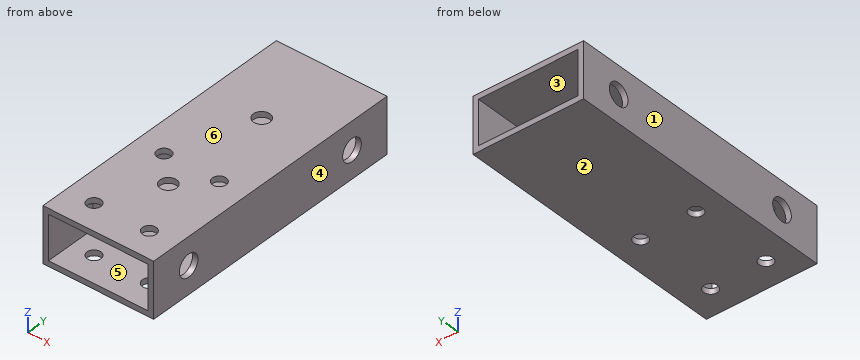
```python
from build123d import *

# Parameters (mm, degrees)
SKICA1_W                 = 40
SKICA1_H                 = 20
SKICA1_W_2               = 36
SKICA1_H_2               = 16
P_IDAT_VYSUNUT_M1_DEPTH  = 100
SKICA2_R                 = 4
ODEBRAT_VYSUNUT_M1_DEPTH = 40
SKETCH1_R                = 2.5
CUT_EXTRUDE1_DEPTH       = 20
SKETCH2_R                = 3
CUT_EXTRUDE2_DEPTH       = 2


with BuildPart() as part:
    # Skica1 → Přidat vysunutím1 (new body)
    with BuildSketch(Plane(origin=(0, 0, 0), x_dir=(1, 0, 0), z_dir=(0, 1, 0))):
        with Locations((20, 10)):
            Rectangle(SKICA1_W, SKICA1_H)
        with Locations((20, 10)):
            Rectangle(SKICA1_W_2, SKICA1_H_2, mode=Mode.SUBTRACT)
    extrude(amount=P_IDAT_VYSUNUT_M1_DEPTH)

    # Skica2 → Odebrat vysunutím1 (cut)
    with BuildSketch(Plane(origin=(40, 0, 0), x_dir=(0, 0, -1), z_dir=(1, 0, 0))):
        with Locations((10, 85)):
            Circle(SKICA2_R)
        with Locations((10, 15)):
            Circle(SKICA2_R)
    extrude(amount=-ODEBRAT_VYSUNUT_M1_DEPTH, mode=Mode.SUBTRACT)

    # Sketch1 → Cut-Extrude1 (cut)
    with BuildSketch(Plane.XY):
        with Locations((10, 10)):
            Circle(SKETCH1_R)
        with Locations((30, 10)):
            Circle(SKETCH1_R)
        with Locations((30, 40)):
            Circle(SKETCH1_R)
        with Locations((10, 40)):
            Circle(SKETCH1_R)
    extrude(amount=-CUT_EXTRUDE1_DEPTH, mode=Mode.SUBTRACT)

    # Sketch2 → Cut-Extrude2 (cut)
    with BuildSketch(Plane.XY):
        with Locations((20, 30)):
            Circle(SKETCH2_R)
        with Locations((20, 70)):
            Circle(SKETCH2_R)
    extrude(amount=-CUT_EXTRUDE2_DEPTH, mode=Mode.SUBTRACT)


solid = part.part
```
Build history of the part. All positions in model axes, mm. Face numbers are marked on the shaded views. A direction names the side the tool comes from. Round coordinates to 2 decimals unless told otherwise and drop trailing zeros. Write each loop counter-clockwise with the first axis right and the second up, starting at its lowest first coordinate (ties: lowest second). Pieces come first, ordered by that corner, then holes.
1) Pin check, flat tips, straight feed: pin 1 (4 mm diameter, centred on x = 10, y = 40, fed in from +Z); pin 2 (5 mm diameter, centred on x = 20, y = 70, fed in from +Z). Stop position of each tip, or through.
2) 3-axis set-ups, long thin cutter, end or side, ignore diameter. For the marked faces 5 and 6: which of +Z, -Z, +X, -X, +Y, -Y reach the whole face in a straight line?
3) Band-saw the part on A-A, the plane z = -5. List the corners of the cut face in (x, y), and give its area (3 significant figures).
4) Drill centre lines: probe 1 along Y at (x, z) = (38.95, -10); probe 2 along X at (y, z) = (37.5, -11.5); probe 3 along Z at (x, y) = (34.5, 90). Where is each one in solid material? Low to high.
5) Mould opens along X. For the marked faces 1, 2, 3 and 4 say: +X half, -X half, draft (parallel to the pull), parting line (faces both ways), or undercut.
6) Band-saw the part on B-B, the plane y = 15. List the corners of the cut face in (x, z), and give its area (3 significant figures).
7) Band-saw the part on C-C, the plane x = 30. List the corners of the cut face in (y, z).
8) Band-saw the part on D-D, the plane x = 20. List the corners of the cut face in (y, z), and give its area (3 significant figures).
Ans:
1. pin 1: passes through
1. pin 2: stops at z = -18
2. face 5: +Y, -Y
2. face 6: +Z, +X, -X, +Y, -Y
3. outline: (0, 0) - (2, 0) - (2, 100) - (0, 100) - close; (38, 0) - (40, 0) - (40, 100) - (38, 100) - close
3. area: 400 mm2
4. probe 1: y = 0 to 11, 19 to 81, 89 to 100
4. probe 2: x = 0 to 2, 38 to 40
4. probe 3: z = -20 to -18, -2 to 0
5. face 1: -X half
5. face 2: draft
5. face 3: undercut
5. face 4: +X half
6. outline: (0, -20) - (40, -20) - (40, -14) - (38, -14) - (38, -18) - (2, -18) - (2, -14) - (0, -14) - close; (0, -6) - (2, -6) - (2, -2) - (38, -2) - (38, -6) - (40, -6) - (40, 0) - (0, 0) - close
6. area: 192 mm2
7. outline: (0, -20) - (7.5, -20) - (7.5, -18) - (0, -18) - close; (0, -2) - (7.5, -2) - (7.5, 0) - (0, 0) - close; (12.5, -20) - (37.5, -20) - (37.5, -18) - (12.5, -18) - close; (12.5, -2) - (37.5, -2) - (37.5, 0) - (12.5, 0) - close; (42.5, -20) - (100, -20) - (100, -18) - (42.5, -18) - close; (42.5, -2) - (100, -2) - (100, 0) - (42.5, 0) - close
8. outline: (0, -20) - (100, -20) - (100, -18) - (0, -18) - close; (0, -2) - (27, -2) - (27, 0) - (0, 0) - close; (33, -2) - (67, -2) - (67, 0) - (33, 0) - close; (73, -2) - (100, -2) - (100, 0) - (73, 0) - close
8. area: 376 mm2
